```python
from build123d import *

# Parameters (mm, degrees)
SKETCH1_W                     = 75
SKETCH1_H                     = 10
BOSS_EXTRUDE1_DEPTH           = 4
M3X0_5_TAPPED_HOLE1_D         = 2.5
CSK_FOR_M3_SFHCS1_D           = 3
CSK_FOR_M3_SFHCS1_CSINK_D     = 5.6
CSK_FOR_M3_SFHCS1_CSINK_ANGLE = 90
CSK_FOR_M3_SFHCS2_D           = 2
CSK_FOR_M3_SFHCS2_CSINK_D     = 4.4
CSK_FOR_M3_SFHCS2_CSINK_ANGLE = 90
M2_5X0_45_TAPPED_HOLE1_D      = 2.05
M2_5X0_45_TAPPED_HOLE1_DEPTH  = 6.35
M2_5X0_45_TAPPED_HOLE1_TIP    = 0.615882135
M2_5X0_45_TAPPED_HOLE2_D      = 2.05
M2_5X0_45_TAPPED_HOLE2_DEPTH  = 6.35
M2_5X0_45_TAPPED_HOLE2_TIP    = 0.615882135


with BuildPart() as part:
    # Sketch1 → Boss-Extrude1 (new body)
    with BuildSketch(Plane.XY.offset(4)):
        Rectangle(SKETCH1_W, SKETCH1_H)
    extrude(amount=-BOSS_EXTRUDE1_DEPTH)

    # M3x0.5 Tapped Hole1 (through all)
    with Locations(Plane(origin=(0, 0, 0), x_dir=(-1, 0, 0), z_dir=(0, 0, -1))):
        with Locations((-13, -2), (13, -2)):
            Hole(M3X0_5_TAPPED_HOLE1_D / 2)

    # CSK for M3 SFHCS1 (through all)
    with Locations(Plane(origin=(0, 0, 0), x_dir=(-1, 0, 0), z_dir=(0, 0, -1))):
        with Locations((-22, -1.5), (20.5, -1.5)):
            CounterSinkHole(CSK_FOR_M3_SFHCS1_D / 2, CSK_FOR_M3_SFHCS1_CSINK_D / 2, counter_sink_angle=CSK_FOR_M3_SFHCS1_CSINK_ANGLE)

    # CSK for M3 SFHCS2 (through all)
    with Locations(Plane(origin=(0, 0, 0), x_dir=(-1, 0, 0), z_dir=(0, 0, -1))):
        with Locations((23.5, 3), (-25, 3)):
            CounterSinkHole(CSK_FOR_M3_SFHCS2_D / 2, CSK_FOR_M3_SFHCS2_CSINK_D / 2, counter_sink_angle=CSK_FOR_M3_SFHCS2_CSINK_ANGLE)

    # M2.5x0.45 Tapped Hole1
    with Locations(Plane(origin=(37.5, 0, 0), x_dir=(0, 0, -1), z_dir=(1, 0, 0))):
        with Locations((-2, 2.5), (-2, -2.5)):
            Hole(M2_5X0_45_TAPPED_HOLE1_D / 2, depth=M2_5X0_45_TAPPED_HOLE1_DEPTH)
            with Locations((0, 0, -(M2_5X0_45_TAPPED_HOLE1_DEPTH + M2_5X0_45_TAPPED_HOLE1_TIP / 2))):  # 118° drill point
                Cone(0, M2_5X0_45_TAPPED_HOLE1_D / 2, M2_5X0_45_TAPPED_HOLE1_TIP, mode=Mode.SUBTRACT)

    # M2.5x0.45 Tapped Hole2
    with Locations(Plane.ZY.offset(37.5)):
        with Locations((2, -2.5), (2, 2.5)):
            Hole(M2_5X0_45_TAPPED_HOLE2_D / 2, depth=M2_5X0_45_TAPPED_HOLE2_DEPTH)
            with Locations((0, 0, -(M2_5X0_45_TAPPED_HOLE2_DEPTH + M2_5X0_45_TAPPED_HOLE2_TIP / 2))):  # 118° drill point
                Cone(0, M2_5X0_45_TAPPED_HOLE2_D / 2, M2_5X0_45_TAPPED_HOLE2_TIP, mode=Mode.SUBTRACT)


solid = part.part
```
The model under review builds one solid part; all positions refer to its coordinate system, in mm. A direction names the side the tool comes from. Round coordinates to 2 decimals unless told otherwise and drop trailing zeros. Order: outer loops, then holes, each group sorted by start corner. A loop starts at its lowest first (then second) coordinate and runs counter-clockwise, first axis right, second up.
Item 1: For pin 1 (3 mm diameter, centred on x = -23.5, y = 3, fed in from -Z); pin 2 (1.5 mm diameter, centred on x = 14, y = 2.5, fed in from -Z); pin 3 (1.8 mm diameter, centred on y = 2.5, z = 2, fed in from -X); pin 4 (3.5 mm diameter, centred on x = -20.5, y = -1.5, fed in from -Z), all flat-tipped, find the tip position at first contact; note any pin that passes through.
Working result:
pin 1: stops at z = 0.7
pin 2: stops at z = 0
pin 3: stops at x = -31.07
pin 4: stops at z = 1.05
Item 2: To check wall thickness, follow probe 1 along Z at (x, y) = (35.5, 2.5) (3 decimals); probe 2 along Y at (x, z) = (-33.5, 2) (3 decimals); probe 3 along X at (y, z) = (-0.5, 0.5). State the ranges of each line that lie inside material, in increasing order.
Working result:
probe 1: z = 0 to 0.975, 3.025 to 4
probe 2: y = -5 to -3.525, -1.475 to 1.475, 3.525 to 5
probe 3: x = -37.5 to -22.57, -18.43 to 19.93, 24.07 to 37.5
Item 3: Draft analysis for pull direction Y (two halves, no side actions). For faces 1 (the flat face through (-1, -5, 2)), 2 (the flat face through (-1, 5, 2)), 3 (the flat face through (-1, 0, 0)), 4 (the conical face through (-30.64, -2.67, 1.96)), state which applies: released by +Y, released by -Y, zero draft, split by the parting line, or undercut.
Working result:
face 1: released by -Y
face 2: released by +Y
face 3: zero draft
face 4: undercut
Item 4: Add section B-B, the plane x = -32.5. State the section outline as (y, z) points (3 decimals).
Working result:
outline: (-5, 0) - (5, 0) - (5, 4) - (-5, 4) - close; hole circle Ø2.05 at (-2.5, 2); hole circle Ø2.05 at (2.5, 2)
Item 5: Add section A-A, the plane x = -20.5. State the section outline as (y, z) points.
Working result:
outline: (-5, 0) - (-4.3, 0) - (-3, 1.3) - (-3, 4) - (-5, 4) - close; (0, 1.3) - (1.3, 0) - (5, 0) - (5, 4) - (0, 4) - close
Item 6: Machinability: for faces 5 (the cylindrical face through (12.079, -1.155, 2.028)), 6 (the cylindrical face through (-34.281, -2.455, 3.024)), 7 (the cylindrical face through (34.281, 1.876, 1.187)), which of the approach directions +Z, -Z, +X, -X, +Y, -Y give a long, thin tool a straight path to every point of the face, cutting with its end or side? Answer none if there is none.
Working result:
face 5: +Z, -Z
face 6: -X
face 7: +X
